The listing builds one solid part. Answer for the finished solid, in the listing's coordinates (mm). A direction names the side the tool comes from. Give positions to 0.01 mm unless a question says otherwise; leave off trailing zeros. Order: outer loops, then holes, each group sorted by start corner. A loop starts at its lowest first (then second) coordinate and runs counter-clockwise, first axis right, second up.
Autodesk Inventor part; units mm, degrees
ref_plane "YZ Plane" through (0, 0, 0) normal (1, 0, 0) x (0, 1, 0)
ref_plane "XZ Plane" through (0, 0, 0) normal (0, 1, 0) x (-1, 0, 0)
ref_plane "XY Plane" through (0, 0, 0) normal (0, 0, 1) x (1, 0, 0)
sketch "Sketch1" plane through (0, 0, 0) normal (0, 0, 1) x (1, 0, 0)
  line L0 (-24.1415, 15.787) -> (24.1415, 15.787)
  line L1 (24.1415, 15.787) -> (24.1415, -15.787)
  line L2 (24.1415, -15.787) -> (-24.1415, -15.787)
  line L3 (-24.1415, -15.787) -> (-24.1415, 15.787)
  point P0 (0, 0)
  dimension "d0" = 31.574
  dimension "d1" = 48.283
  dimension "d2" = 24.1415
  dimension "d3" = 15.787
extrude "Extrusion1" add sketch "Sketch1" against normal blind 26.136
fillet "Fillet1" radius 8.5 5 edges at (0, -15.787, 0) (24.1415, 0, 0) (-24.1415, 0, 0) (-24.1415, -15.787, -13.068) (24.1415, -15.787, -13.068)
shell "Shell1" thickness 2.5 removed faces 2 at (5.2138, 15.787, -17.424) at (-5.2138, 5.2623, -26.136)
sketch "Sketch2" plane through (-24.1415, -7.287, -8.5) normal (-1, 0, 0) x (0, 0, 1)
  line L0 (0, 23.074) -> (-17.636, 23.074)
  line L1 (-17.636, 23.074) -> (-17.636, 0)
  line L2 (-17.636, -0.926) -> (-0.636, -0.926)
  line L3 (-0.636, -0.926) -> (-0.636, 23.074)
  line L4 (-0.636, 23.074) -> (-17.636, 23.074)
  line L5 (-17.636, 23.074) -> (-17.636, -0.926)
  point P0 (8.5, 7.287)
  dimension "d8" = 17
  dimension "d9" = 24
extrude "Extrusion2" cut sketch "Sketch2" against normal through all
sketch "Sketch3" plane through (-15.6415, 15.787, 0) normal (0, 1, 0) x (1, 0, 0)
  line L0 (39.783, 8.5) -> (39.783, 9.136)
  line L1 (39.783, 9.136) -> (34.783, 9.136)
  line L2 (34.783, 9.136) -> (14.783, 26.136)
  line L3 (0, 26.136) -> (31.283, 26.136)
  line L4 (39.783, 9.136) -> (39.783, 26.136)
  line L5 (39.783, 26.136) -> (14.783, 26.136)
  point P0 (15.6415, 0)
  dimension "d12" = 5
  dimension "d13" = 20
extrude "Extrusion3" cut sketch "Sketch3" against normal through all
fillet "Fillet2" radius 4 6 edges at (-22.8303, -8.213, -26.136) (19.1415, -13.5967, -9.136) (-22.8303, -8.213, -9.136) (-22.8915, 15.787, -9.136) (22.8915, 15.787, -9.136) (-0.8585, -14.537, -26.136)
sketch "Sketch4" plane through (0, 0, 0) normal (0, 0, 1) x (1, 0, 0)
  line L0 (0.2618, -15.787) -> (-2.3288, -15.787)
  line L1 (0.2618, -15.787) -> (15.6415, -15.787)
  line L2 (-15.6415, -15.787) -> (15.6415, -15.787)
  line L3 (-15.6415, -15.787) -> (-2.3288, -15.787)
  line L4 (-24.1415, 11.787) -> (-24.1415, 13.9511)
  line L5 (-24.1415, 11.787) -> (-24.1415, -4.213)
  line L6 (-24.1415, -4.213) -> (-24.1415, -7.287)
  line L7 (-24.1415, 13.9511) -> (-24.1415, -7.287)
  point P0 (0, 0)
  point P1 (3.4645, 2.911)
  dimension "d17" = 27.606
  dimension "d18" = 18.698
hole "Hole1" at (3.4645, 2.911, 0) direction (0, 0, -1) diameter 12.8 end through all
sketch "Sketch5" plane through (-15.6415, -15.787, -8.5) normal (0, -1, 0) x (1, 0, 0)
  line L0 (-8.5, -2.0766) -> (-8.5, -0.636)
  line L1 (12.706, 8.5) -> (25.506, 8.5)
  line L2 (0, 8.5) -> (31.283, 8.5)
  line L3 (31.283, 8.5) -> (0, 8.5)
  point P0 (15.6415, 8.5)
  point P1 (7.163, -7.48)
  dimension "d26" = 15.663
  dimension "d27" = 15.98
hole "Hole2" at (-8.4785, -15.787, -15.98) direction (0, 1, 0) diameter 8 end through all
properties part number "314-08" material "Steel"
1) Find section C-C (z = -15.98). Write down the section's boundary in (x, y), then the cut area to 3 significant figures.
Geometry says:
outline: (-24.09, -8.21) arc R8.5 ccw to (-15.64, -15.79) - (-12.48, -15.79) - (-12.48, -13.29) - (-15.64, -13.29) arc R6 cw to (-21.57, -8.21) - close; (-4.48, -15.79) - (11.09, -15.79) - (11.09, -13.29) - (-4.48, -13.29) - close
area: 73.0 mm2
2) Given P1, Ø2, axis at x = -8, y = -9, coming from the -Z side; P2, Ø6.5, axis at x = -8.48, z = -15.98, coming from the -Y side; P3, Ø3, axis at x = -23, z = -20, coming from the +Y side; P4, Ø1, axis at y = -1, z = -4.5, coming from the +X side, each flat-ended and moving along its own axis, determine where each tip first touches the part or whether it passes through.
Geometry says:
P1: stops at z = -3.15
P2: passes through
P3: stops at y = -8.21
P4: stops at x = 23.39
3) For a pull along Y with two mould halves and no side action, classify faces 5 (the cylindrical face through (1.542, -3.193, -1.268)), 6 (the flat face through (-4, 4, 0)), 7 (the flat face through (0, -15.787, -15)) as +Y half, -Y half, draft (parallel to the pull), parting line (faces both ways), or undercut.
Geometry says:
face 5: undercut
face 6: draft
face 7: -Y half
4) Straight lines are drawn through the part: probe 1 along Z at (x, y) = (-3, -6.5); probe 2 along Y at (x, z) = (-15, -19.5); probe 3 along X at (y, z) = (-14.4, -15.98). For each, find the intervals that lie inside material, in ascending order.
Geometry says:
probe 1: z = -2.5 to 0
probe 2: y = -15.79 to -13.29
probe 3: x = -20.3 to -12.48, -4.48 to 11.09
5) A tool of negligible diameter and unlimited length cuts with its end or side. For faces 1 (the flat face through (23, -1, -9.136)), 2 (the flat face through (-23, -8.213, -18)), 3 (the cylindrical face through (18.508, -12.558, -9.378)), 4 (the flat face through (-13, -14, -26.136)), from which of +Z, -Z, +X, -X, +Y, -Y can it reach the whole face along a straight path? Write none if from no direction.
Geometry says:
face 1: -Z, +X, +Y, -Y
face 2: -Z, +X, -X, +Y
face 3: -Z, +Y
face 4: -Z, +X, -X, +Y, -Y
6) Find section A-A (x = -5). Write down the section's boundary in (y, z).
Geometry says:
outline: (-15.79, -26.14) - (-13.29, -26.14) - (-13.29, -17.95) - (-15.79, -17.95) - close; (-15.79, -14.01) - (-13.29, -14.01) - (-13.29, -8.5) arc R6 cw to (-7.29, -2.5) - (15.79, -2.5) - (15.79, 0) - (-7.29, 0) arc R8.5 ccw to (-15.79, -8.5) - close
7) Find section D-D (x = 11). Write down the section's boundary in (y, z).
Geometry says:
outline: (-15.79, -16.06) - (-13.29, -16.06) - (-13.29, -8.5) arc R6 cw to (-7.29, -2.5) - (15.79, -2.5) - (15.79, 0) - (-7.29, 0) arc R8.5 ccw to (-15.79, -8.5) - close
8) Find section B-B (y = 3). Write down the section's boundary in (x, z), then the cut area to 3 significant figures.
Geometry says:
outline: (-24.14, -9.14) - (-21.64, -9.14) - (-21.64, -8.5) arc R6 cw to (-15.64, -2.5) - (-2.93, -2.5) - (-2.93, 0) - (-15.64, 0) arc R8.5 ccw to (-24.14, -8.5) - close; (9.86, -2.5) - (15.64, -2.5) arc R6 cw to (21.64, -8.5) - (21.64, -9.14) - (24.14, -9.14) - (24.14, -8.5) arc R8.5 ccw to (15.64, 0) - (9.86, 0) - close
area: 106 mm2
